Design review of the part built by this model. Coordinates are the model's own, in mm. Give positions to 0.01 mm unless a question says otherwise; leave off trailing zeros. Write each loop counter-clockwise with the first axis right and the second up, starting at its lowest first coordinate (ties: lowest second). Pieces come first, ordered by that corner, then holes.
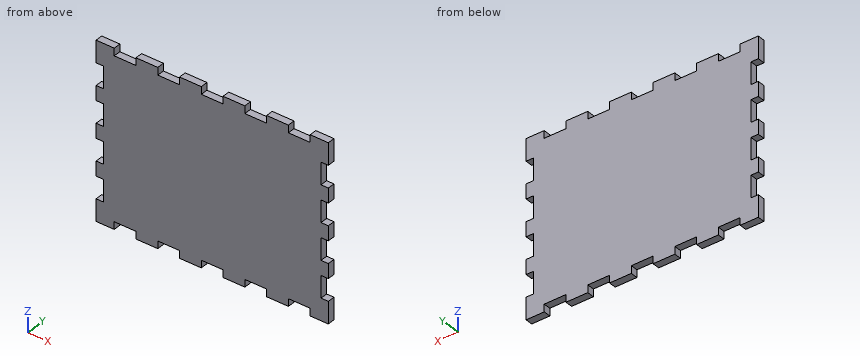
```python
from build123d import *

# Parameters (mm, degrees)
SKETCH1_W               = 203.2
SKETCH1_H               = 152.4
BOSS_EXTRUDE1_DEPTH     = 3.175
SKETCH2_W               = 19.05
SKETCH2_H               = 6.477
CUT_EXTRUDE1_DEPTH      = 128.158650905
LPATTERN1_COUNT         = 5
LPATTERN1_PITCH         = 38.1
MIRROR1_COPY_1_SKETCH_W = 19.05
MIRROR1_COPY_1_SKETCH_H = 6.477
MIRROR1_COPY_1_DEPTH    = 128.158650905
MIRROR1_COPY_2_SKETCH_W = 19.05
MIRROR1_COPY_2_SKETCH_H = 6.477
MIRROR1_COPY_2_DEPTH    = 128.158650905
MIRROR1_COPY_3_SKETCH_W = 19.05
MIRROR1_COPY_3_SKETCH_H = 6.477
MIRROR1_COPY_3_DEPTH    = 128.158650905
MIRROR1_COPY_4_SKETCH_W = 19.05
MIRROR1_COPY_4_SKETCH_H = 6.477
MIRROR1_COPY_4_DEPTH    = 128.158650905
SKETCH3_W               = 6.35
SKETCH3_H               = 19.05
CUT_EXTRUDE2_DEPTH      = 128.158650905
LPATTERN2_COUNT         = 4
LPATTERN2_PITCH         = 31.75
MIRROR2_COPY_1_SKETCH_W = 6.35
MIRROR2_COPY_1_SKETCH_H = 19.05
MIRROR2_COPY_1_DEPTH    = 128.158650905
MIRROR2_COPY_2_SKETCH_W = 6.35
MIRROR2_COPY_2_SKETCH_H = 19.05
MIRROR2_COPY_2_DEPTH    = 128.158650905
MIRROR2_COPY_3_SKETCH_W = 6.35
MIRROR2_COPY_3_SKETCH_H = 19.05
MIRROR2_COPY_3_DEPTH    = 128.158650905


with BuildPart() as part:
    # Sketch1 → Boss-Extrude1 (new, symmetric)
    with BuildSketch(Plane(origin=(0, 0, 0), x_dir=(1, 0, 0), z_dir=(0, 1, 0))):
        Rectangle(SKETCH1_W, SKETCH1_H)
    extrude(amount=BOSS_EXTRUDE1_DEPTH, both=True)

    # Sketch2 → Cut-Extrude1 (cut, through all)
    with BuildSketch(Plane(origin=(0, 3.175, 0), x_dir=(1, 0, 0), z_dir=(0, 1, 0))):
        with Locations((76.2, 72.9615)):
            Rectangle(SKETCH2_W, SKETCH2_H)
    cut_extrude1 = extrude(amount=-CUT_EXTRUDE1_DEPTH, mode=Mode.SUBTRACT)

    # LPattern1: Cut-Extrude1 ×5
    with Locations(*[(-i * LPATTERN1_PITCH, 0, 0) for i in range(1, LPATTERN1_COUNT)]):
        add(cut_extrude1, mode=Mode.SUBTRACT)

    # Mirror1: Cut-Extrude1 across plane
    add(cut_extrude1.mirror(Plane.XY), mode=Mode.SUBTRACT)

    # Mirror1 copy 1 sketch → Mirror1 copy 1 (cut, through all)
    with BuildSketch(Plane(origin=(-38.1, 3.175, 0), x_dir=(1, 0, 0), z_dir=(0, 1, 0))):
        with Locations((76.2, -72.9615)):
            Rectangle(MIRROR1_COPY_1_SKETCH_W, MIRROR1_COPY_1_SKETCH_H)
    extrude(amount=-MIRROR1_COPY_1_DEPTH, mode=Mode.SUBTRACT)

    # Mirror1 copy 2 sketch → Mirror1 copy 2 (cut, through all)
    with BuildSketch(Plane(origin=(-76.2, 3.175, 0), x_dir=(1, 0, 0), z_dir=(0, 1, 0))):
        with Locations((76.2, -72.9615)):
            Rectangle(MIRROR1_COPY_2_SKETCH_W, MIRROR1_COPY_2_SKETCH_H)
    extrude(amount=-MIRROR1_COPY_2_DEPTH, mode=Mode.SUBTRACT)

    # Mirror1 copy 3 sketch → Mirror1 copy 3 (cut, through all)
    with BuildSketch(Plane(origin=(-114.3, 3.175, 0), x_dir=(1, 0, 0), z_dir=(0, 1, 0))):
        with Locations((76.2, -72.9615)):
            Rectangle(MIRROR1_COPY_3_SKETCH_W, MIRROR1_COPY_3_SKETCH_H)
    extrude(amount=-MIRROR1_COPY_3_DEPTH, mode=Mode.SUBTRACT)

    # Mirror1 copy 4 sketch → Mirror1 copy 4 (cut, through all)
    with BuildSketch(Plane(origin=(-152.4, 3.175, 0), x_dir=(1, 0, 0), z_dir=(0, 1, 0))):
        with Locations((76.2, -72.9615)):
            Rectangle(MIRROR1_COPY_4_SKETCH_W, MIRROR1_COPY_4_SKETCH_H)
    extrude(amount=-MIRROR1_COPY_4_DEPTH, mode=Mode.SUBTRACT)

    # Sketch3 → Cut-Extrude2 (cut, through all)
    with BuildSketch(Plane(origin=(0, 3.175, 0), x_dir=(1, 0, 0), z_dir=(0, 1, 0))):
        with Locations((-98.425, 47.625)):
            Rectangle(SKETCH3_W, SKETCH3_H)
    cut_extrude2 = extrude(amount=-CUT_EXTRUDE2_DEPTH, mode=Mode.SUBTRACT)

    # LPattern2: Cut-Extrude2 ×4
    with Locations(*[(0, 0, i * LPATTERN2_PITCH) for i in range(1, LPATTERN2_COUNT)]):
        add(cut_extrude2, mode=Mode.SUBTRACT)

    # Mirror2: Cut-Extrude2 across plane
    add(cut_extrude2.mirror(Plane(origin=(0, 0, 0), x_dir=(0, 0, 1), z_dir=(1, 0, 0))), mode=Mode.SUBTRACT)

    # Mirror2 copy 1 sketch → Mirror2 copy 1 (cut, through all)
    with BuildSketch(Plane(origin=(0, 3.175, 31.75), x_dir=(-1, 0, 0), z_dir=(0, 1, 0))):
        with Locations((-98.425, -47.625)):
            Rectangle(MIRROR2_COPY_1_SKETCH_W, MIRROR2_COPY_1_SKETCH_H)
    extrude(amount=-MIRROR2_COPY_1_DEPTH, mode=Mode.SUBTRACT)

    # Mirror2 copy 2 sketch → Mirror2 copy 2 (cut, through all)
    with BuildSketch(Plane(origin=(0, 3.175, 63.5), x_dir=(-1, 0, 0), z_dir=(0, 1, 0))):
        with Locations((-98.425, -47.625)):
            Rectangle(MIRROR2_COPY_2_SKETCH_W, MIRROR2_COPY_2_SKETCH_H)
    extrude(amount=-MIRROR2_COPY_2_DEPTH, mode=Mode.SUBTRACT)

    # Mirror2 copy 3 sketch → Mirror2 copy 3 (cut, through all)
    with BuildSketch(Plane(origin=(0, 3.175, 95.25), x_dir=(-1, 0, 0), z_dir=(0, 1, 0))):
        with Locations((-98.425, -47.625)):
            Rectangle(MIRROR2_COPY_3_SKETCH_W, MIRROR2_COPY_3_SKETCH_H)
    extrude(amount=-MIRROR2_COPY_3_DEPTH, mode=Mode.SUBTRACT)


solid = part.part
```
(1) To check wall thickness, follow L1, parallel to X at y = -1.25, z = -48; L2, parallel to Z at x = -8, y = -0.5. State the ranges of each line that lie inside material, in increasing order.
Resolved:
L1: x = -95.25 to 95.25
L2: z = -69.72 to 69.72
(2) Consider section B-B, the plane x = 37.5. Give the boundary of the cut face in (y, z) (3 decimals), then the cut area to 3 significant figures.
Resolved:
outline: (-3.175, -69.723) - (3.175, -69.723) - (3.175, 69.723) - (-3.175, 69.723) - close
area: 885 mm2
(3) Clearance check with flat-ended pins moving along their axes: P1, Ø1.9, axis at y = 0, z = -15.5, coming from the -X side; P2, Ø1.9, axis at y = -1, z = 48, coming from the +X side. State where each tip first meets the part, or that it passes through.
Resolved:
P1: stops at x = -95.25
P2: stops at x = 95.25
(4) Consider section A-A, the plane z = -21. Give the boundary of the cut face in (x, y) (3 decimals).
Resolved:
outline: (-95.25, -3.175) - (95.25, -3.175) - (95.25, 3.175) - (-95.25, 3.175) - close
